```python
from build123d import *

# Parameters (mm, degrees)
EXTRUDE_1_DEPTH        = 34
SKETCH_2_R             = 18
EXTRUDE_2_DEPTH        = 28.5
SKETCH_3_R             = 11
EXTRUDE_3_DEPTH        = 2
SKETCH_4_R             = 4
EXTRUDE_4_DEPTH        = 18
SKETCH_5_W             = 8.09428643
SKETCH_5_H             = 13.450799509
CUT_EXTRUDE_1_DEPTH    = 15
SKETCH_6_R             = 1
CUT_EXTRUDE_2_DEPTH    = 5
HOLE_WIZARD_M3_1_D     = 2.5
HOLE_WIZARD_M3_1_DEPTH = 7.5
HOLE_WIZARD_M3_1_TIP   = 0.751075774


with BuildPart() as part:
    # 草图1 → 凸台-拉伸1 (new body)
    with BuildSketch(Plane.XY):
        Polygon((-21.15, 16.15), (-16.15, 21.15), (16.15, 21.15), (21.15, 16.15), (21.15, -16.15), (16.15, -21.15), (-16.15, -21.15), (-21.15, -16.15), align=None)
    extrude(amount=EXTRUDE_1_DEPTH)

    # 草图2 → 凸台-拉伸2 (add)
    with BuildSketch(Plane.XY.offset(34)):
        Circle(SKETCH_2_R)
    extrude(amount=EXTRUDE_2_DEPTH)

    # 草图3 → 凸台-拉伸3 (add)
    with BuildSketch(Plane.XY.offset(62.5)):
        Circle(SKETCH_3_R)
    extrude(amount=EXTRUDE_3_DEPTH)

    # 草图4 → 凸台-拉伸4 (add)
    with BuildSketch(Plane.XY.offset(64.5)):
        Circle(SKETCH_4_R)
    extrude(amount=EXTRUDE_4_DEPTH)

    # 草图5 → 切除-拉伸1 (cut)
    with BuildSketch(Plane.XY.offset(82.5)):
        with Locations((-7.047143215, -1.347451383)):
            Rectangle(SKETCH_5_W, SKETCH_5_H)
    extrude(amount=-CUT_EXTRUDE_1_DEPTH, mode=Mode.SUBTRACT)

    # 草图6 → 切除-拉伸2 (cut)
    with BuildSketch(Plane.XY.offset(62.5)):
        with Locations((-10.606601718, 10.606601718)):
            Circle(SKETCH_6_R)
        with Locations((10.606601718, 10.606601718)):
            Circle(SKETCH_6_R)
        with Locations((-10.606601718, -10.606601718)):
            Circle(SKETCH_6_R)
        with Locations((10.606601718, -10.606601718)):
            Circle(SKETCH_6_R)
    extrude(amount=-CUT_EXTRUDE_2_DEPTH, mode=Mode.SUBTRACT)

    # M3 螺纹孔1
    with Locations(Plane.XY.offset(62.5)):
        with Locations((-10.606601718, 10.606601718), (10.606601718, 10.606601718), (-10.606601718, -10.606601718), (10.606601718, -10.606601718)):
            Hole(HOLE_WIZARD_M3_1_D / 2, depth=HOLE_WIZARD_M3_1_DEPTH)
            with Locations((0, 0, -(HOLE_WIZARD_M3_1_DEPTH + HOLE_WIZARD_M3_1_TIP / 2))):  # 118° drill point
                Cone(0, HOLE_WIZARD_M3_1_D / 2, HOLE_WIZARD_M3_1_TIP, mode=Mode.SUBTRACT)


solid = part.part
```
Check sheet for the modelled part. Datum: model origin and axes. Units: mm. A direction names the side the tool comes from. Round coordinates to 2 decimals unless told otherwise and drop trailing zeros. Order: outer loops, then holes, each group sorted by start corner. A loop starts at its lowest first (then second) coordinate and runs counter-clockwise, first axis right, second up. Notation, with made-up numbers: (85.5, 57) -> (134.5, 57) arc R30 ccw to (134.5, 91) -> close; hole circle Ø4 at (35, 7). An arc over 180 degrees is marked (long way). Use CSV: the item, a comma, the result in double quotes.
(1) Material ranges on line 1 along Z through (x, y) = (-17, -1); line 2 along X through (y, z) = (-11.5, 59); line 3 along Z through (x, y) = (-18, -10), recorded low to high. Write a range as from..to.
Worked out:
line 1,"0..62.5"
line 2,"-13.85..-11.48, -9.73..9.73, 11.48..13.85"
line 3,"0..34"
(2) Depth check by flat-ended pin: pin 1 (0.5 mm diameter, centred on x = -3.5, y = 0, fed in from +Z); pin 2 (10 mm diameter, centred on x = 9, y = -11.5, fed in from +Z); pin 3 (2.5 mm diameter, centred on y = 0.5, z = 72, fed in from -X); pin 4 (2 mm diameter, centred on x = 10.61, y = 10.61, fed in from -Z). Enter the tip coordinate at first touch or a pass-through.
Worked out:
pin 1,"z = 67.5"
pin 2,"z = 64.5"
pin 3,"x = -3"
pin 4,"z = 0"
(3) Cross-section at D-D (x = -17). Record the boundary of the cut face in (y, z), and give its area (3 significant figures).
Worked out:
outline,"(-20.3, 0) -> (20.3, 0) -> (20.3, 34) -> (5.92, 34) -> (5.92, 62.5) -> (-5.92, 62.5) -> (-5.92, 34) -> (-20.3, 34) -> close"
area,"1,720 mm²"
(4) Tool access check on faces 4 (the face through (-3, 0, 75)), 5 (the face through (0, -21.15, 17)), 6 (the face through (10.878, -11.827, 58.698)). Record the directions out of +Z, -Z, +X, -X, +Y, -Y that give a thin tool (end or side, any length) a straight path to the whole face; none if there is none.
Worked out:
face 4,"+Z, -X, +Y, -Y"
face 5,"+Z, -Z, +X, -X, -Y"
face 6,"+Z"
(5) Draft check along X on faces 1 (the face through (0, -5, 64.5)), 2 (the face through (-10.77, -10.46, 54.38)), 3 (the face through (-18.7, 18.6, 16.8)). Enter one of: pulls with the +X half, pulls with the -X half, needs draft (parallel to the pull), parting line crosses it, or undercut.
Worked out:
face 1,"needs draft"
face 2,"undercut"
face 3,"pulls with the -X half"
(6) Cross-section at A-A (x = 0). Record the boundary of the cut face in (y, z), and give its area (3 significant figures).
Worked out:
outline,"(-21.15, 0) -> (21.15, 0) -> (21.15, 34) -> (18, 34) -> (18, 62.5) -> (11, 62.5) -> (11, 64.5) -> (4, 64.5) -> (4, 82.5) -> (-4, 82.5) -> (-4, 64.5) -> (-11, 64.5) -> (-11, 62.5) -> (-18, 62.5) -> (-18, 34) -> (-21.15, 34) -> close"
area,"2,650 mm²"
(7) Cross-section at C-C (y = 0). Record the boundary of the cut face in (x, z), and give its area (3 significant figures).
Worked out:
outline,"(-21.15, 0) -> (21.15, 0) -> (21.15, 34) -> (18, 34) -> (18, 62.5) -> (11, 62.5) -> (11, 64.5) -> (4, 64.5) -> (4, 82.5) -> (-3, 82.5) -> (-3, 67.5) -> (-4, 67.5) -> (-4, 64.5) -> (-11, 64.5) -> (-11, 62.5) -> (-18, 62.5) -> (-18, 34) -> (-21.15, 34) -> close"
area,"2,640 mm²"
(8) Cross-section at B-B (z = 21). Record the boundary of the cut face in (x, y), and give its area (3 significant figures).
Worked out:
outline,"(-21.15, -16.15) -> (-16.15, -21.15) -> (16.15, -21.15) -> (21.15, -16.15) -> (21.15, 16.15) -> (16.15, 21.15) -> (-16.15, 21.15) -> (-21.15, 16.15) -> close"
area,"1,740 mm²"
